```python
from build123d import *

# Parameters (mm, degrees)
F0_W     = 100
F0_H     = 500
F1_DEPTH = 100
F2_W     = 100
F2_H     = 70
F3_DEPTH = 10
F4_SCALE = 0.07


with BuildPart() as f1:
    # F0 (on Front) → F1 (new body)
    with BuildSketch(Plane.XZ):
        with Locations((50, 250)):
            Rectangle(F0_W, F0_H)
    extrude(amount=F1_DEPTH)

    # F2 (on face) → F3 (cut)
    with BuildSketch(Plane.XY.offset(500)):
        with Locations((50, -65)):
            Rectangle(F2_W, F2_H)
    extrude(amount=-F3_DEPTH, mode=Mode.SUBTRACT)


with BuildPart() as f1_1:
    # F4: moved
    add(f1.part.scale(F4_SCALE))


solid = f1_1.part
```
Verification items for the finished model (mm, model axes). A direction names the side the tool comes from. Round coordinates to 2 decimals unless told otherwise and drop trailing zeros. Order: outer loops, then holes, each group sorted by start corner. A loop starts at its lowest first (then second) coordinate and runs counter-clockwise, first axis right, second up. Notation, with made-up numbers: (-7.75, 22.25) - (37.25, 22.25) arc R25 ccw to (37.25, 36.25) - close; hole circle Ø11 at (4.25, 14.25). An arc over 180 degrees is marked (long way). Use CSV: the item, a comma, the result in double quotes. Start each with the question number.
1) Thickness scan on L1, parallel to Z at x = 3.25, y = -2.5. Record the ranges inside material, lowest first.
2) Section check A-A, the plane y = -5.5. Record the cut outline in (x, z).
3) Go/stop test with flat-tipped pins: P1, Ø1, axis at y = -1.5, z = 6, coming from the -X side; P2, Ø2.5, axis at x = 3.5, y = -4, coming from the +Z side. Record where each tip stops, or that it passes through.
4) Access from +Z, -Z, +X, -X, +Y, -Y to the whole of each face (thin tool, end or side, straight path). Record for faces 1 (the flat face through (3, -1, 35)), 2 (the flat face through (3, -5, 34.3)).
Answers:
1,L1,"z = 0 to 34.3"
2,outline,"(0, 0) - (7, 0) - (7, 34.3) - (0, 34.3) - close"
3,P1,"stops at x = 0"
3,P2,"stops at z = 34.3"
4,face 1,"+Z, +X, -X, +Y, -Y"
4,face 2,"+Z, +X, -X, -Y"
